```python
from build123d import *

# Parameters (mm, degrees)
F0_W     = 50
F0_H     = 50
F1_DEPTH = 100
F3_D     = 6.6
F4_R     = 20.2206931271
F4_R_2   = 20.8160873388
F5_DEPTH = 150
F6_R     = 57.5
F7_DEPTH = 100


with BuildPart() as f1:
    # F0 (on Front) → F1 (new body, symmetric)
    with BuildSketch(Plane.XZ):
        with Locations((25, 25)):
            Rectangle(F0_W, F0_H)
    extrude(amount=F1_DEPTH, both=True)

    # F3 (through all)
    with Locations(Plane.XY.offset(50)):
        with Locations((25, 99.4929849688), (24.9502013015, 33.496488903), (25.2753126699, -35.7510662615), (26.9008440388, -91.3441732113)):
            Hole(F3_D / 2)

    # F4 (on face) → F5 (join)
    with BuildSketch(Plane.YZ.offset(50)):
        with Locations((-56.6662251949, 23.0115242302)):
            Circle(F4_R)
        with Locations((55.072888732, 25.1332446933)):
            Circle(F4_R_2)
    extrude(amount=F5_DEPTH)

    # F6 (on Front) → F7 (join, symmetric)
    with BuildSketch(Plane.XZ):
        with Locations((199.8447626829, 25.3131054342)):
            Circle(F6_R)
    extrude(amount=F7_DEPTH, both=True)

    # F9 (on offset) → F10 (revolve, cut)
    with BuildSketch(Plane(origin=(200, 0, 0), x_dir=(0, -1, 0), z_dir=(-1, 0, 0))):
        Polygon((-105.5897921324, 24.3519060314), (100.8795276284, 24.3519060314), (101.4911159873, 24.6927142143), (105.1713102595, 25.4731605558), (104.8070022361, 65.9113094268), (79.0776162995, 65.679512918), (79.2472240509, 46.8530719335), (-62.0798177726, 45.5798540268), (-62.2608959675, 65.679512918), (-105.5897921324, 65.2891620994), align=None)
    revolve(axis=Axis((200, 2.355132252, 24.3519060314), (0, 1, 0)), mode=Mode.SUBTRACT)


solid = f1.part
```
Part model, mm, in its own coordinate system. A direction names the side the tool comes from. Coordinates: 2 decimals unless noted, no trailing zeros. Write each loop counter-clockwise with the first axis right and the second up, starting at its lowest first coordinate (ties: lowest second). Pieces come first, ordered by that corner, then holes.
Item 1: Slice it at C-C (z = 34). Count the separate pieces of the cut face and the enclosed holes in it, and give its area (3 significant figures).
Item 2: Probe line 1 (Y direction, x = 115, z = 24); line 2 (X direction, y = -8, z = 8); line 3 (Y direction, x = 225.5, z = 15). List the from-to ranges inside material, lowest first.
Item 3: Slice it at D-D (y = 53). Write the cut outline in (x, z), and give its area (3 significant figures).
Item 4: Slice it at A-A (y = -17). Write the cut outline in (x, z).
Item 5: Which spindle directions (+Z, -Z, +X, -X, +Y, -Y) get a long thin tool onto all of the face, cutting with end or side? Do faces 4 (the face through (23.427, 30.569, 24.65)), 5 (the face through (159.823, 81.395, 15.43)), 6 (the face through (223.22, -79.24, 21.3)), 7 (the face through (25, -1, 0)). Say none if no direction does.
Item 6: Mould opens along X. For faces 1 (the face through (23.5, -32.97, 24.65)), 2 (the face through (212, 100, 64)), 3 (the face through (0, -1, 25)) say: released by +X, released by -X, zero draft, split by the parting line, or undercut.
Item 7: Slice it at B-B (x = 139). Write the cut outline in (y, z), and give its area (3 significant figures).
Item 8: Pin check, flat tips, straight feed: pin 1 (10 mm diameter, centred on y = 15.5, z = -18.5, fed in from +X); pin 2 (25 mm diameter, centred on x = 19, y = -31.5, fed in from +Z); pin 3 (1.5 mm diameter, centred on y = 75.5, z = -13.5, fed in from -X). Stop position of each tip, or through.
Results found:
1. separate pieces: 2
1. enclosed holes: 4
1. area: 29,000 mm2
2. line 1: y = -76.86 to -36.47, 34.29 to 75.86
2. line 2: x = 0 to 50, 145.01 to 185.49, 214.51 to 254.68
2. line 3: y = -79.21 to 62.13
3. outline: (0, 0) - (50, 0) - (50, 4.42) - (146.27, 4.42) arc R57.5 ccw (long way) to (146.14, 45.85) - (50, 45.85) - (50, 50) - (0, 50) - close; hole circle Ø42.62 at (200, 24.35)
3. area: 15,300 mm2
4. outline: (0, 0) - (50, 0) - (50, 50) - (0, 50) - close; circle Ø115 at (199.84, 25.31); hole circle Ø43.88 at (200, 24.35)
5. face 4: +Z, -Z
5. face 5: none
5. face 6: -Y
5. face 7: -Z, -X, +Y, -Y
6. face 1: undercut
6. face 2: zero draft
6. face 3: released by -X
7. outline: circle Ø40.44 at (-56.67, 23.01); circle Ø41.63 at (55.07, 25.13)
7. area: 2,650 mm2
8. pin 1: stops at x = 242.27
8. pin 2: stops at z = 50
8. pin 3: stops at x = 156.75
